The figure shows three views and two pictorial views of one solid part (mm, origin at its lowest corner). Answer the questions. A direction names the side the tool comes from. Round coordinates to 2 decimals unless told otherwise and drop trailing zeros. Order: outer loops, then holes, each group sorted by start corner. A loop starts at its lowest first (then second) coordinate and runs counter-clockwise, first axis right, second up. Notation, with made-up numbers: (80.25, -23) - (110.25, -23) arc R20 cw to (110.25, 2) - close; hole circle Ø8 at (22.5, 33). An arc over 180 degrees is marked (long way). Answer as a JSON object with one key per item and string values. Group by question number.
Q1. A tool of negligible diameter and unlimited length cuts with its end or side. For the marked faces 4 and 5, from which of +Z, -Z, +X, -X, +Y, -Y can it reach the whole face along a straight path? Write none if from no direction.
Q2. A cutting plane is placed at C-C on y = 4.25. Determine the outline of the cut face in (x, z).
Q3. Given pin 1 Ø2 at (y, z) = (7, 7) entering from -X; pin 2 Ø1.5 at (y, z) = (6, 4) entering from +X, each flat-ended and moving along its own axis, determine where each tip first touches the part or whether it passes through.
Q4. The mould has two halves that part along X. Classify the marked faces 1, 2 and 3: pulls with the +X half, pulls with the -X half, needs draft (parallel to the pull), parting line crosses it, or undercut.
Q5. Consider line 1 (X direction, y = 5, z = 6.25); line 2 (X direction, y = 4.25, z = 5.25); line 3 (Y direction, x = 8, z = 1.5) (1 decimal). Determine where each line is inside the solid, lowest interval first.
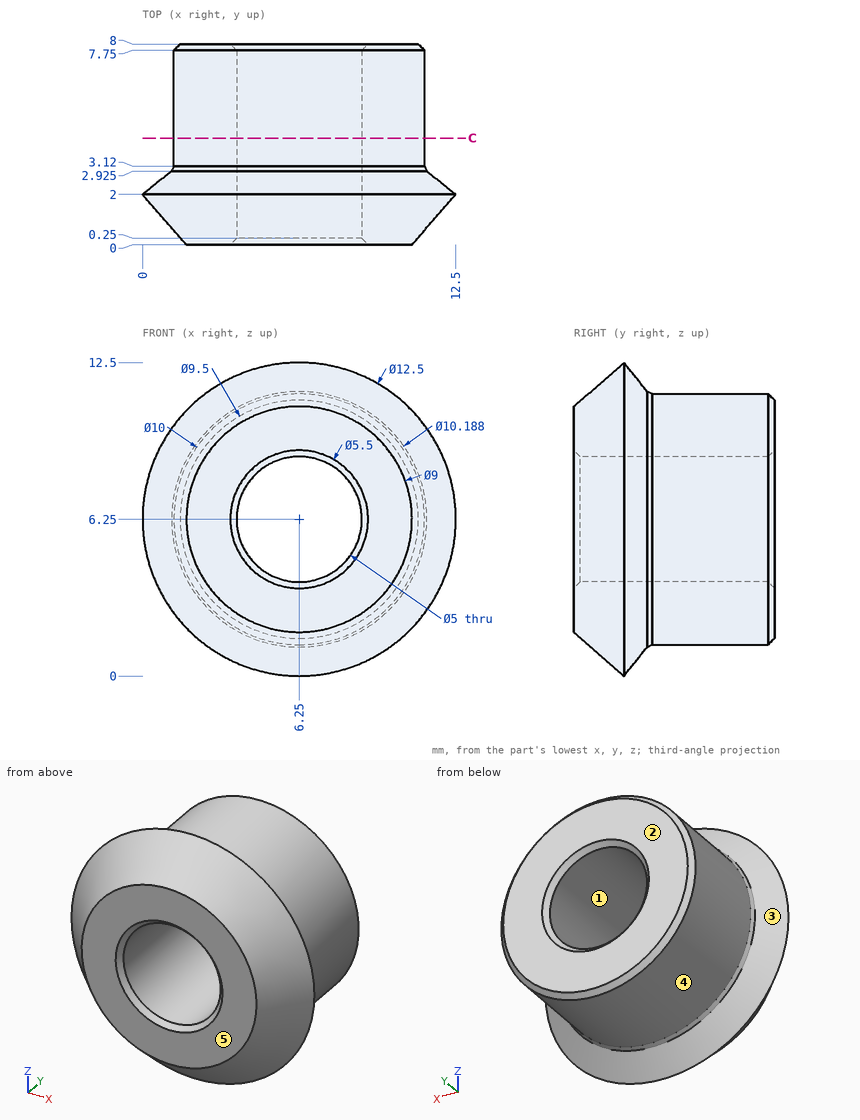
Result set:
{
 "1": {"face 4": "+Y", "face 5": "+Z, -Z, +X, -X, -Y"},
 "2": {"outline": "circle Ø10 at (6.25, 6.25); hole circle Ø5 at (6.25, 6.25)"},
 "3": {"pin 1": "stops at x = 1.25", "pin 2": "stops at x = 11.02"},
 "4": {"face 1": "undercut", "face 2": "needs draft", "face 3": "parting line crosses it"},
 "5": {"line 1": "x = 1.25 to 3.75, 8.75 to 11.25", "line 2": "x = 1.35 to 3.96, 8.54 to 11.15", "line 3": "y = 0.6 to 3"}
}
